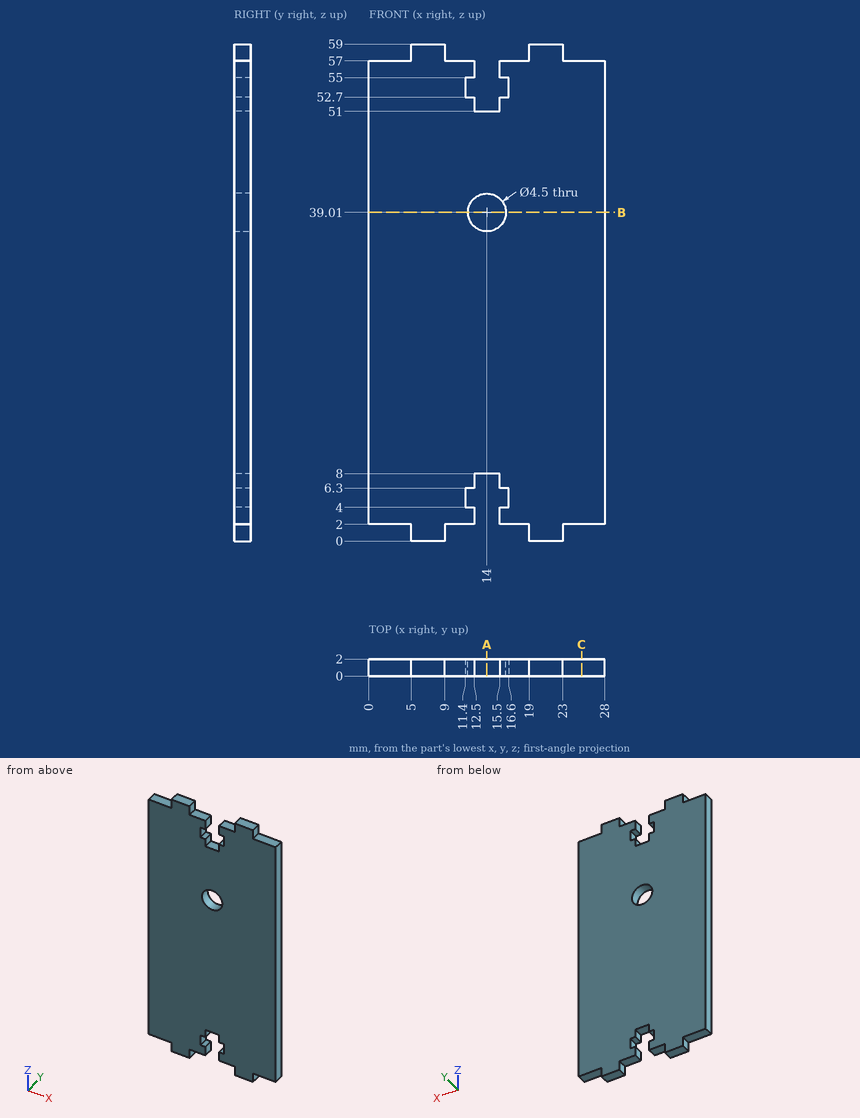
Geometry check sheet. Reference: drawing and pictorial views, mm from the part's lowest x, y, z. Round coordinates to 2 decimals unless told otherwise and drop trailing zeros. Loops run counter-clockwise (first coordinate to the right, second up) from the corner with the lowest first, then second, coordinate; pieces in that order, holes last. Notation, with made-up numbers: (23.25, 22) - (37.25, 22) arc R8 ccw to (37.25, 29) - close; hole circle Ø5 at (-20.75, -7). An arc over 180 degrees is marked (long way). Use a Markdown table: item, result.
Q1. Cross-section at C-C on x = 25.25. Record the cut outline in (y, z).
Solutions:
| item | result |
|---|---|
| outline | (0, 2) - (2, 2) - (2, 57) - (0, 57) - close |
Q2. Go/stop test with flat-tipped pins: P1, Ø0.9, axis at x = 12, y = 1, coming from the -Z side; P2, Ø3.5, axis at x = 14, z = 39.01, coming from the -Y side; P3, Ø1.2, axis at x = 16, y = 1, coming from the +Z side; P4, Ø0.6, axis at y = 1, z = 1, coming from the +X side. Record where each tip stops, or that it passes through.
Solutions:
| item | result |
|---|---|
| P1 | stops at z = 2 |
| P2 | passes through |
| P3 | stops at z = 57 |
| P4 | stops at x = 23 |
Q3. Material ranges on line 1 (Z direction, x = 11.5, y = 1.45); line 2 (X direction, y = 1.2, z = 52); line 3 (X direction, y = 1.25, z = 39.01), recorded low to high.
Solutions:
| item | result |
|---|---|
| line 1 | z = 2 to 4, 6.3 to 52.7, 55 to 57 |
| line 2 | x = 0 to 12.5, 15.5 to 28 |
| line 3 | x = 0 to 11.75, 16.25 to 28 |
Q4. Cross-section at B-B on z = 39.01. Record the cut outline in (x, y), plus the area to 3 significant figures.
Solutions:
| item | result |
|---|---|
| outline | (0, 0) - (11.75, 0) - (11.75, 2) - (0, 2) - close; (16.25, 0) - (28, 0) - (28, 2) - (16.25, 2) - close |
| area | 47.0 mm2 |
Q5. Cross-section at A-A on x = 14. Record the cut outline in (y, z).
Solutions:
| item | result |
|---|---|
| outline | (0, 8) - (2, 8) - (2, 36.76) - (0, 36.76) - close; (0, 41.26) - (2, 41.26) - (2, 51) - (0, 51) - close |
